For this review, take the finished solid that the model builds, in its own axes (mm). A direction names the side the tool comes from. Round coordinates to 2 decimals unless told otherwise and drop trailing zeros. Order: outer loops, then holes, each group sorted by start corner. A loop starts at its lowest first (then second) coordinate and runs counter-clockwise, first axis right, second up.
Autodesk Inventor part; units mm, degrees
ref_plane "YZ Plane" through (0, 0, 0) normal (1, 0, 0) x (0, 1, 0)
ref_plane "XZ Plane" through (0, 0, 0) normal (0, 1, 0) x (-1, 0, 0)
ref_plane "XY Plane" through (0, 0, 0) normal (0, 0, 1) x (1, 0, 0)
sketch "Sketch1" plane through (0, 0, 0) normal (0, 0, 1) x (1, 0, 0)
  circle A0 centre (0, 0) radius 50.8
  dimension "d0" = 101.6
extrude "Extrusion1" add sketch "Sketch1" along normal blind 63.5
sketch "Sketch2" plane through (0, 0, 63.5) normal (0, 0, 1) x (1, 0, 0)
  circle A0 centre (0, 0) radius 50.8
  circle A1 centre (0, 0) radius 9.525
  dimension "d5" = 19.05
extrude "Extrusion2" add sketch "Sketch2" along normal blind 15.875 and the other way blind 76.2 contours A1
sketch "Sketch3" plane through (0, 0, 79.375) normal (0, 0, 1) x (1, 0, 0)
  line L0 (-15.875, -55.5625) -> (79.375, -55.5625)
  line L1 (79.375, -55.5625) -> (79.375, 14.2875)
  line L2 (79.375, 14.2875) -> (-15.875, 14.2875)
  line L3 (-15.875, 14.2875) -> (-15.875, -55.5625)
  dimension "d11" = 95.25
  dimension "d13" = 69.85
extrude "Extrusion3" add sketch "Sketch3" along normal blind 1.524
sketch "Sketch4" plane through (0, 0, 79.375) normal (0, 0, -1) x (-1, 0, 0)
  line L0 (15.875, -55.5625) -> (-79.375, -55.5625)
  line L1 (15.875, 14.2875) -> (15.875, -55.5625)
  line L2 (-79.375, -55.5625) -> (15.875, -55.5625)
  line L3 (15.875, -55.5625) -> (15.875, -54.0385)
  line L4 (15.875, -54.0385) -> (-79.375, -54.0385)
  line L5 (-79.375, -54.0385) -> (-79.375, -55.5625)
  point P0 (-79.375, 14.2875)
  dimension "d16" = 1.524
  dimension "d47" = 69.85
  dimension "d48" = 95.25
extrude "Extrusion4" add sketch "Sketch4" along normal blind 88.9
sketch "Sketch5" plane through (0, 0, -9.525) normal (0, 0, -1) x (-1, 0, 0)
  line L0 (-79.375, -55.5625) -> (15.875, -55.5625)
  line L1 (15.875, -55.5625) -> (15.875, 14.2875)
  line L2 (15.875, 14.2875) -> (-79.375, 14.2875)
  line L3 (-79.375, 14.2875) -> (-79.375, -55.5625)
  point P0 (0, 0)
extrude "Extrusion5" add sketch "Sketch5" along normal blind 1.524
sketch "Sketch6" plane through (0, 0, 80.899) normal (0, 0, 1) x (1, 0, 0)
  circle A0 centre (66.2655, 4.5181) radius 4.7625
  point P0 (0, 0)
  dimension "d21" = 9.525
extrude "Extrusion6" add sketch "Sketch6" along normal blind 12.7 and the other way blind 95.25
sketch "Sketch7" plane through (66.2655, 4.5181, 93.599) normal (0, 0, 1) x (1, 0, 0)
  line L0 (-5.1033, 11.8715) -> (159.8746, 107.1215)
  line L1 (159.8746, 107.1215) -> (172.5746, 85.1244)
  line L2 (172.5746, 85.1244) -> (7.5967, -10.1256)
  line L3 (7.5967, -10.1256) -> (-5.1033, 11.8715)
  line L4 (0, 0) -> (168.275, 0) construction
  point P0 (-66.2655, -4.5181)
  dimension "d29" = 25.4
  dimension "d30" = 190.5
  dimension "d40" = 30
extrude "Extrusion7" add sketch "Sketch7" along normal blind 6.35
sketch "Sketch8" plane through (66.2655, 4.5181, 99.949) normal (0, 0, 1) x (1, 0, 0)
  line L0 (172.5746, 85.1244) -> (159.8746, 107.1215)
  circle A0 centre (155.226, 89.773) radius 6.35
  point P0 (-66.2655, -4.5181)
  dimension "d43" = 12.7
  dimension "d44" = 12.7
extrude "Extrusion8" add sketch "Sketch8" along normal blind 101.6
sketch "Sketch9" plane through (-15.875, -55.5625, 80.899) normal (0, -1, 0) x (1, 0, 0)
  line L0 (0, 0) -> (0, -91.948)
  line L1 (95.25, -91.948) -> (0, -91.948)
  circle A0 centre (12.7, -45.974) radius 4.7625
  circle A1 centre (82.55, -45.974) radius 4.7625
  point P0 (15.875, -80.899)
  dimension "d49" = 91.948
  dimension "d50" = 95.25
  dimension "d51" = 9.525
  dimension "d52" = 12.7
  dimension "d55" = 69.85
hole "Hole1" at (66.675, -55.5625, 34.925) at (-3.175, -55.5625, 34.925) direction (0, 1, 0) diameter 9.525 depth 2.54 tip angle 118
properties part number "0winch"
(1) Wall thickness on L1, parallel to Z at x = 122.5, y = 46.5; L2, parallel to Z at x = -34.5, y = -32; L3, parallel to Y at x = 26.5, z = 57: over which ranges is each line inside the solid? List them lowest first.
(2) Add section C-C on y = -14.5. Give the boundary of the cut face in (x, z) (3 decimals).
(3) Add section D-D on z = 134. Give the boundary of the cut face in (x, y).
(4) Tool access review of faces 4 (the face through (-3.384, -54.79, 39.683)), 5 (the face through (31, -54.038, 36)), 6 (the face through (70.665, 2.694, 35.547)): name each direction out of +Z, -Z, +X, -X, +Y, -Y from which nothing blocks a thin tool from reaching the whole face with its end or side.
(5) Add section B-B on z = 24. Give the boundary of the cut face in (x, y) (1 decimal).
(6) Draft analysis for pull direction X (two halves, no side actions). For faces 1 (the face through (70.665, 6.342, 87.16)), 2 (the face through (-7.559, -5.796, -4.696)), 3 (the face through (221, 94, 201.549)), state which applies: pulls with the +X half, pulls with the -X half, needs draft (parallel to the pull), parting line crosses it, or undercut.
(7) Clearance check with flat-ended pins moving along their axes: P1, Ø0.5, axis at x = 38.5, z = 80.5, coming from the +Y side; P2, Ø8, axis at x = 29, z = 71.5, coming from the +Y side; P3, Ø7.5, axis at x = 66.675, z = 34.925, coming from the -Y side. State where each tip first meets the part, or that it passes through.
(8) Add section A-A on x = 23.5. Give the boundary of the cut face in (y, z) (1 decimal).
Here are the results:
1. L1: z = 93.6 to 99.95
1. L2: z = 0 to 63.5
1. L3: y = -55.56 to -54.04, -43.34 to 43.34
2. outline: (-48.687, 0) - (48.687, 0) - (48.687, 63.5) - (-48.687, 63.5) - close; (-15.875, -11.049) - (79.375, -11.049) - (79.375, -9.525) - (-15.875, -9.525) - close; (-15.875, 79.375) - (79.375, 79.375) - (79.375, 80.899) - (-15.875, 80.899) - close
3. outline: circle Ø12.7 at (221.49, 94.29)
4. face 4: -Y
4. face 5: +X, -X
4. face 6: none
5. outline: circle Ø101.6 at (0, 0); (-15.9, -55.6) - (79.4, -55.6) - (79.4, -54) - (-15.9, -54) - close; circle Ø9.5 at (66.3, 4.5)
6. face 1: parting line crosses it
6. face 2: undercut
6. face 3: needs draft
7. P1: stops at y = 14.29
7. P2: stops at y = -54.04
7. P3: stops at y = -0.24
8. outline: (-55.6, -11) - (14.3, -11) - (14.3, -9.5) - (-54, -9.5) - (-54, 79.4) - (14.3, 79.4) - (14.3, 80.9) - (-55.6, 80.9) - close; (-45, 0) - (45, 0) - (45, 63.5) - (-45, 63.5) - close
